```python
from build123d import *

# Parameters (mm, degrees)
SKETCH1_W           = 42
SKETCH1_H           = 42
BOSS_EXTRUDE1_DEPTH = 34
SKETCH2_R           = 2.5
BOSS_EXTRUDE2_DEPTH = 25
SKETCH3_R           = 11
BOSS_EXTRUDE3_DEPTH = 2
SKETCH4_W           = 1
SKETCH4_H           = 6
CUT_EXTRUDE1_DEPTH  = 15


with BuildPart() as part:
    # Sketch1 → Boss-Extrude1 (new body)
    with BuildSketch(Plane.XY):
        Rectangle(SKETCH1_W, SKETCH1_H)
    extrude(amount=-BOSS_EXTRUDE1_DEPTH)

    # Sketch2 → Boss-Extrude2 (add)
    with BuildSketch(Plane.XY):
        Circle(SKETCH2_R)
    extrude(amount=BOSS_EXTRUDE2_DEPTH)

    # Sketch3 → Boss-Extrude3 (add)
    with BuildSketch(Plane.XY):
        with Locations(Location((0, 0, 0), (0, 0, 180))):
            Circle(SKETCH3_R)
    extrude(amount=BOSS_EXTRUDE3_DEPTH)

    # Sketch4 → Cut-Extrude1 (cut)
    with BuildSketch(Plane.XY.offset(23)):
        with Locations((2.5, 0)):
            Rectangle(SKETCH4_W, SKETCH4_H)
    extrude(amount=-CUT_EXTRUDE1_DEPTH, mode=Mode.SUBTRACT)


solid = part.part
```
The listing builds one solid part. Answer for the finished solid, in the listing's coordinates (mm). A direction names the side the tool comes from. Round coordinates to 2 decimals unless told otherwise and drop trailing zeros. Loops run counter-clockwise (first coordinate to the right, second up) from the corner with the lowest first, then second, coordinate; pieces in that order, holes last. Notation, with made-up numbers: (-8.5, 84.25) - (-2.5, 84.25) arc R25 ccw to (-2.5, 113.25) - close; hole circle Ø9 at (-20.75, -16.5). An arc over 180 degrees is marked (long way). Use one line per item in the form item = value. Start each with the question number.
1. The part is cut by section D-D on x = 9.5. Determine the outline of the cut face in (y, z), then the cut area to 3 significant figures.
2. Consider line 1 (Z direction, x = -5, y = 11); line 2 (Z direction, x = 7.5, y = -8); line 3 (Y direction, x = 0.5, z = 11.5). Determine where each line is inside the solid, lowest interval first. Write a range as [from, to].
3. For a pull along Z with two mould halves and no side action, classify faces 1 (the face through (0, 0, 25)), 2 (the face through (0, 0, -34)), 3 (the face through (2, 0, 16)) as pulls with the +Z half, pulls with the -Z half, needs draft (parallel to the pull), parting line crosses it, or undercut.
4. The part is cut by section C-C on z = 15.5. Determine the outline of the cut face in (x, y), then the cut area to 3 significant figures.
5. A tool of negligible diameter and unlimited length cuts with its end or side. For faces 4 (the face through (21, 0, -17)), 5 (the face through (-2.5, 0.1, 13.3)), from which of +Z, -Z, +X, -X, +Y, -Y can it reach the whole face along a straight path? Write none if from no direction.
6. The part is cut by section B-B on y = 0. Determine the outline of the cut face in (x, z).
7. Given pin 1 Ø1 at (y, z) = (-9, 2) entering from +X; pin 2 Ø10 at (x, y) = (5.5, -13.5) entering from +Z; pin 3 Ø2.5 at (y, z) = (0, 18.5) entering from +X; pin 4 Ø17.5 at (x, y) = (-2, -4) entering from +Z, each flat-ended and moving along its own axis, determine where each tip first touches the part or whether it passes through.
8. The part is cut by section A-A on x = 0. Determine the outline of the cut face in (y, z), then the cut area to 3 significant figures.
Geometry check:
q1.outline = (-21, -34) - (21, -34) - (21, 0) - (5.55, 0) - (5.55, 2) - (-5.55, 2) - (-5.55, 0) - (-21, 0) - close
q1.area = 1,450 mm^2
q2.line_1 = [-34, 0]
q2.line_2 = [-34, 2]
q2.line_3 = [-2.45, 2.45]
q3.face_1 = pulls with the +Z half
q3.face_2 = pulls with the -Z half
q3.face_3 = undercut
q4.outline = (2, -1.5) - (2, 1.5) arc R2.5 ccw (long way) to start
q4.area = 18.6 mm^2
q5.face_4 = +Z, -Z, +X, +Y, -Y
q5.face_5 = +Z
q6.outline = (-21, -34) - (21, -34) - (21, 0) - (11, 0) - (11, 2) - (2.5, 2) - (2.5, 8) - (2, 8) - (2, 23) - (2.5, 23) - (2.5, 25) - (-2.5, 25) - (-2.5, 2) - (-11, 2) - (-11, 0) - (-21, 0) - close
q7.pin_1 = 6.98
q7.pin_2 = 2
q7.pin_3 = 2
q7.pin_4 = 25
q8.outline = (-21, -34) - (21, -34) - (21, 0) - (11, 0) - (11, 2) - (2.5, 2) - (2.5, 25) - (-2.5, 25) - (-2.5, 2) - (-11, 2) - (-11, 0) - (-21, 0) - close
q8.area = 1,590 mm^2
